Model file for the job. Use its own axes, mm. A direction names the side the tool comes from. Round coordinates to 2 decimals unless told otherwise and drop trailing zeros. Order: outer loops, then holes, each group sorted by start corner. A loop starts at its lowest first (then second) coordinate and runs counter-clockwise, first axis right, second up. Notation, with made-up numbers: (28.5, 52.25) -> (61.5, 52.25) arc R26 ccw to (61.5, 84.25) -> close; hole circle Ø3 at (-23.75, -29). An arc over 180 degrees is marked (long way). Put each result on its own line as item: value. Start each with the question number.
Q1. Pull direction X, two halves, no side cores. Call faces 1 (the face through (-6.848, 4, 3)), 2 (the face through (0, -1.964, 3)), 3 (the face through (0, 15.536, 3)): released by +X, released by -X, zero draft, split by the parting line, or undercut.
Q2. Cut at A-A, the plane y = -3. List the corners of the cut face in (x, z).
Q3. Flat gauge pin, fed straight in: P1, Ø5.5, axis at x = 0.15, y = 8.54, coming from the +Z side (3 decimals). Where does the tip first touch, or does it go through?
Q4. Cut at C-C, the plane z = 3.2. List the corners of the cut face in (x, y).
Q5. Cut at D-D, the plane y = 6. List the corners of the cut face in (x, z), and give its area (3 significant figures).
Q6. Cut at B-B, the plane x = 3.25. List the corners of the cut face in (y, z).
Q7. Probe L1, parallel to X at y = -4, z = 3.1; L2, parallel to Y at x = 1.75, z = 3.55; L3, parallel to Y at x = 1, z = 1.8. List the from-to ranges inside material, lowest first.
Q8. 3-axis set-ups, long thin cutter, end or side, ignore diameter. For faces 4 (the face through (-3.848, -3, 3)), 5 (the face through (0, -7.964, 3)): which of +Z, -Z, +X, -X, +Y, -Y reach the whole face in a straight line?
from build123d import *

# Parameters (mm, degrees)
SKETCH1_W           = 14
SKETCH1_H           = 23.5
SKETCH1_R           = 3.5
SKETCH1_W_2         = 8
SKETCH1_H_2         = 3
BOSS_EXTRUDE2_DEPTH = 6


with BuildPart() as part:
    # Sketch1 → Boss-Extrude2 (new body)
    with BuildSketch(Plane.XY):
        with Locations((0.151915527, 3.785637599)):
            Rectangle(SKETCH1_W, SKETCH1_H)
        with Locations((0.151915527, 8.535637599)):
            Circle(SKETCH1_R, mode=Mode.SUBTRACT)
        with Locations((0.151915527, -3.464362401)):
            Rectangle(SKETCH1_W_2, SKETCH1_H_2, mode=Mode.SUBTRACT)
    extrude(amount=BOSS_EXTRUDE2_DEPTH)


solid = part.part
Ans:
1. face 1: released by -X
1. face 2: undercut
1. face 3: zero draft
2. outline: (-6.85, 0) -> (-3.85, 0) -> (-3.85, 6) -> (-6.85, 6) -> close; (4.15, 0) -> (7.15, 0) -> (7.15, 6) -> (4.15, 6) -> close
3. P1: passes through
4. outline: (-6.85, -7.96) -> (7.15, -7.96) -> (7.15, 15.54) -> (-6.85, 15.54) -> close; hole (-3.85, -4.96) -> (4.15, -4.96) -> (4.15, -1.96) -> (-3.85, -1.96) -> close; hole circle Ø7 at (0.15, 8.54)
5. outline: (-6.85, 0) -> (-2.26, 0) -> (-2.26, 6) -> (-6.85, 6) -> close; (2.56, 0) -> (7.15, 0) -> (7.15, 6) -> (2.56, 6) -> close
5. area: 55.0 mm^2
6. outline: (-7.96, 0) -> (-4.96, 0) -> (-4.96, 6) -> (-7.96, 6) -> close; (-1.96, 0) -> (6.91, 0) -> (6.91, 6) -> (-1.96, 6) -> close; (10.16, 0) -> (15.54, 0) -> (15.54, 6) -> (10.16, 6) -> close
7. L1: x = -6.85 to -3.85, 4.15 to 7.15
7. L2: y = -7.96 to -4.96, -1.96 to 5.42, 11.65 to 15.54
7. L3: y = -7.96 to -4.96, -1.96 to 5.14, 11.93 to 15.54
8. face 4: +Z, -Z
8. face 5: +Z, -Z, +X, -X, -Y
